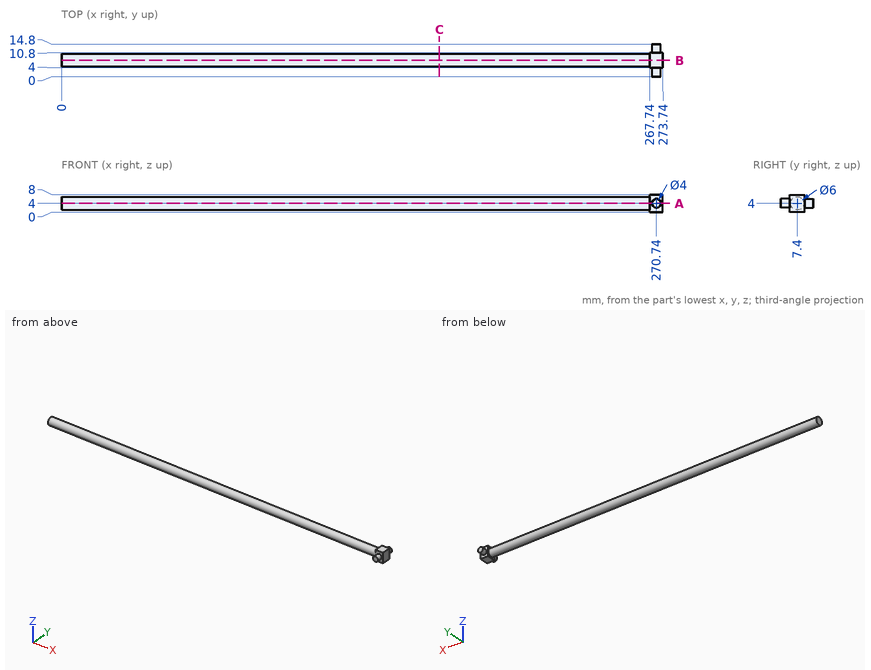
Input: dimensioned drawing with shaded views. Units: mm. Origin: part minimum x, y, z. Give positions to 0.01 mm unless a question says otherwise; leave off trailing zeros. Order: outer loops, then holes, each group sorted by start corner. A loop starts at its lowest first (then second) coordinate and runs counter-clockwise, first axis right, second up. Notation, with made-up numbers: (38, -34) -> (83, -34) arc R8 cw to (83, -25) -> close; hole circle Ø9 at (3.5, -3). An arc over 180 degrees is marked (long way). Use one line per item in the form item = value.
1) Section C-C, the plane x = 172. Return loops of the section in (y, z).
Response values:
outline = circle Ø6 at (7.4, 4)
2) Line query: probe 1 along X at (y, z) = (6.75, 7.25); probe 2 along X at (y, z) = (11.25, 4.25); probe 3 along Z at (x, y) = (27.5, 9.5). Output: solid intervals per line, ascending.
Response values:
probe_1 = 267.74 to 273.74
probe_2 = 268.76 to 272.72
probe_3 = 1.86 to 6.14
3) Section B-B, the plane y = 7.4. Return loops of the section in (x, z).
Response values:
outline = (0, 1) -> (267.74, 1) -> (267.74, 0) -> (273.74, 0) -> (273.74, 8) -> (267.74, 8) -> (267.74, 7) -> (0, 7) -> close
4) Section A-A, the plane z = 4. Return loops of the section in (x, y).
Response values:
outline = (0, 4.4) -> (267.74, 4.4) -> (267.74, 4) -> (268.74, 4) -> (268.74, 0) -> (272.74, 0) -> (272.74, 4) -> (273.74, 4) -> (273.74, 10.8) -> (272.74, 10.8) -> (272.74, 14.8) -> (268.74, 14.8) -> (268.74, 10.8) -> (267.74, 10.8) -> (267.74, 10.4) -> (0, 10.4) -> close
5) First-contact query: pin 1 Ø4 at (x, z) = (29.5, 3.5) entering from +Y; pin 2 Ø4 at (x, y) = (128, 11) entering from -Z; pin 3 Ø1.5 at (x, y) = (144, 7.5) entering from +Z. Flat tips, straight axial feed; report the tip coordinate or a pass-through.
Response values:
pin_1 = 10.4
pin_2 = 1.46
pin_3 = 7
